```python
from build123d import *

# Parameters (mm, degrees)
SKETCH047_R          = 0.8
POCKET027_DEPTH      = 6.3010001
POCKET027_DEPTH_BACK = 3.0010001
POCKET028_DEPTH      = 6.3010001
POCKET028_DEPTH_BACK = 3.0010001
POCKET030_DEPTH      = 123.0422530554
POCKET030_DEPTH_BACK = 119.7422530554


with BuildPart() as part:
    # Sketch046 → AdditiveLoft section 0
    with BuildSketch(Plane.YZ.offset(-15)):
        with BuildLine():
            Line((-19.35, 3), (19.35, 3))
            ThreePointArc((21.0820508076, 2), (20.35, 2.7320508076), (19.35, 3))
            Line((21.0820508076, 2), (21.35, 1.5358983849))
            Line((21.35, 1.5358983849), (21.35, -6.3))
            Line((21.35, -6.3), (19.35, -6.3))
            Line((19.35, 1), (19.35, -6.3))
            Line((-19.35, 1), (19.35, 1))
            Line((-19.35, -6.3), (-19.35, 1))
            Line((-19.35, -6.3), (-21.35, -6.3))
            Line((-21.35, -6.3), (-21.35, 1.5358983849))
            Line((-21.0820508076, 2), (-21.35, 1.5358983849))
            ThreePointArc((-19.35, 3), (-20.35, 2.7320508076), (-21.0820508076, 2))
        make_face()
    # Sketch058 → AdditiveLoft section 1
    with BuildSketch(Plane.YZ.offset(15)):
        with BuildLine():
            Line((-22.6, 3), (22.6, 3))
            ThreePointArc((24.3320508076, 2), (23.6, 2.7320508076), (22.6, 3))
            Line((24.3320508076, 2), (24.6, 1.5358983849))
            Line((24.6, 1.5358983849), (24.6, -6.3))
            Line((24.6, -6.3), (22.6, -6.3))
            Line((22.6, 1), (22.6, -6.3))
            Line((-22.6, 1), (22.6, 1))
            Line((-22.6, -6.3), (-22.6, 1))
            Line((-22.6, -6.3), (-24.6, -6.3))
            Line((-24.6, -6.3), (-24.6, 1.5358983849))
            Line((-24.3320508076, 2), (-24.6, 1.5358983849))
            ThreePointArc((-22.6, 3), (-23.6, 2.7320508076), (-24.3320508076, 2))
        make_face()
    loft()

    # Sketch047 → Pocket027 (cut, two sides)
    with BuildSketch(Plane.XY) as pocket027_sk:
        with Locations((7.9, 7.9)):
            Circle(SKETCH047_R)
        with Locations((-7.9, 7.9)):
            Circle(SKETCH047_R)
        with Locations((-7.9, -7.9)):
            Circle(SKETCH047_R)
        with Locations((7.9, -7.9)):
            Circle(SKETCH047_R)
    extrude(amount=-POCKET027_DEPTH, mode=Mode.SUBTRACT)
    extrude(pocket027_sk.sketch, amount=POCKET027_DEPTH_BACK, mode=Mode.SUBTRACT)

    # Sketch048 → Pocket028 (cut, two sides)
    with BuildSketch(Plane.XY) as pocket028_sk:
        Polygon((9, 5), (16, 7.5477916399), (16, -7.5477916399), (9, -5), align=None)
    extrude(amount=-POCKET028_DEPTH, mode=Mode.SUBTRACT)
    extrude(pocket028_sk.sketch, amount=POCKET028_DEPTH_BACK, mode=Mode.SUBTRACT)

    # Sketch050 → Pocket030 (cut, two sides)
    with BuildSketch(Plane.XY) as pocket030_sk:
        with BuildLine():
            Line((8.3, 30), (18.3, 30))
            Line((18.3, 30), (18.3, 17.3))
            Line((12, 17.3), (18.3, 17.3))
            ThreePointArc((8.3, 21), (9.3837049096, 18.3837049096), (12, 17.3))
            Line((8.3, 21), (8.3, 30))
        make_face()
    pocket030 = extrude(amount=-POCKET030_DEPTH, mode=Mode.SUBTRACT) + extrude(pocket030_sk.sketch, amount=POCKET030_DEPTH_BACK, mode=Mode.SUBTRACT)

    # Mirrored011: Pocket030 across XZ
    add(pocket030.mirror(Plane.XZ), mode=Mode.SUBTRACT)


solid = part.part
```
Work out the finished part from the listing and answer in its coordinate system (mm). A direction names the side the tool comes from. Give positions to 0.01 mm unless a question says otherwise; leave off trailing zeros. Order: outer loops, then holes, each group sorted by start corner. A loop starts at its lowest first (then second) coordinate and runs counter-clockwise, first axis right, second up. Notation, with made-up numbers: M -30,29 L -21,29 A31 ccw -21,58 Z; hole C 75.25,11.25 d11. An arc over 180 degrees is marked long. Return JSON: item names as keys, results as strings.
1) Straight lines are drawn through the part: line 1 along X through (y, z) = (-7.9, 1.5); line 2 along Y through (x, z) = (7.9, 1.85); line 3 along Y through (x, z) = (7.9, 2.15). For each, find the intervals that lie inside material, in ascending order. Write a range as [from, to].
Resolved:
{"line 1": "[-15, -8.7], [-7.1, 7.1], [8.7, 15]", "line 2": "[-23.65, -8.7], [-7.1, 7.1], [8.7, 23.65]", "line 3": "[-23.47, -8.7], [-7.1, 7.1], [8.7, 23.47]"}
2) Each of these flat-tipped pins is pushed along its axis until it touches: pin 1 (1.8 mm diameter, centred on x = 7.9, y = -7.9, fed in from +Z); pin 2 (2 mm diameter, centred on x = -10.5, z = -4, fed in from -Y); pin 3 (2.5 mm diameter, centred on y = 22, z = -3.5, fed in from +X); pin 4 (5 mm diameter, centred on x = 5.5, y = -8, fed in from -Z). Where does it stop, or does it pass through?
Resolved:
{"pin 1": "z = 3", "pin 2": "y = -21.95", "pin 3": "x = 8.3", "pin 4": "z = 1"}
3) For a pull along X with two mould halves and no side action, classify faces 5 (the flat face through (12.042, -6.107, 1.986)), 6 (the flat face through (-15, -0.5, 1.4)), 7 (the cylindrical face through (7.27, 7.41, 1.99)) as +X half, -X half, draft (parallel to the pull), parting line (faces both ways), or undercut.
Resolved:
{"face 5": "+X half", "face 6": "-X half", "face 7": "undercut"}
4) A tool of negligible diameter and unlimited length cuts with its end or side. For faces 1 (the flat face through (8.3, -23, -2)), 2 (the flat face through (11.958, 6.077, 1.986)), 3 (the flat face through (-3.19, 20.63, -2.7)), 4 (the flat face through (13, 17.3, 2)), from which of +Z, -Z, +X, -X, +Y, -Y can it reach the whole face along a straight path? Write none if from no direction.
Resolved:
{"face 1": "+Z, -Z, +X, -Y", "face 2": "+Z, -Z, +X", "face 3": "-Z, +X", "face 4": "+Z, -Z, +X, +Y"}
5) Section B-B, the plane y = -7.9 is taken. Give the number of separate pieces and of enclosed holes in the cut face, plus the area to 3 significant figures.
Resolved:
{"separate pieces": "3", "enclosed holes": "0", "area": "53.6 mm^2"}
6) Section A-A, the plane z = -2.5 is taken. Write down the section's boundary in (x, y), plus the area to 3 significant figures.
Resolved:
{"outline": "M -15,-21.35 L 8.3,-23.87 L 8.3,-21.87 L -15,-19.35 Z; M -15,19.35 L 8.3,21.87 L 8.3,23.87 L -15,21.35 Z", "area": "93.2 mm^2"}
